Input: part model. Units: mm. Frame: model coordinates. Face numbers are marked on the shaded views. A direction names the side the tool comes from. Round coordinates to 2 decimals unless told otherwise and drop trailing zeros. Loops run counter-clockwise (first coordinate to the right, second up) from the corner with the lowest first, then second, coordinate; pieces in that order, holes last.
1) Section C-C, the plane y = 14.75. Return loops of the section in (x, z).
2) Section D-D, the plane z = 3.75. Return loops of the section in (x, y), and give its area (4 significant figures).
3) First-contact query: pin 1 (2.5 mm diameter, centred on x = 19.5, y = 4.5, fed in from +Z); pin 2 (8 mm diameter, centred on x = 25.5, y = 22, fed in from -Z); pin 3 (9.5 mm diameter, centred on x = 53.5, y = 13.5, fed in from +Z). Flat tips, straight axial feed; report the tip coordinate or a pass-through.
4) Section B-B, the plane x = 29. Return loops of the section in (y, z), and give its area (4 significant figures).
5) Draft query along X for the marked faces 1, 2 and 3. Return one class per face: pulls with the +X half, pulls with the -X half, needs draft (parallel to the pull), parting line crosses it, or undercut.
6) Section A-A, the plane z = 7.25. Return loops of the section in (x, y), and give its area (3 significant figures).
7) Access query for the marked faces 4, 5 and 6. Directions: +Z, -Z, +X, -X, +Y, -Y. A direction counts if a zero-diameter tool reaches every point of the face in a straight line with its end or side. Return the directions, or none.
8) Ray query, line 1 along Y through (x, z) = (57.5, 2.25); line 2 along Y through (x, z) = (41, 3.25); line 3 along X through (y, z) = (18.25, 4.5). Return the intervals inside material, ascending.
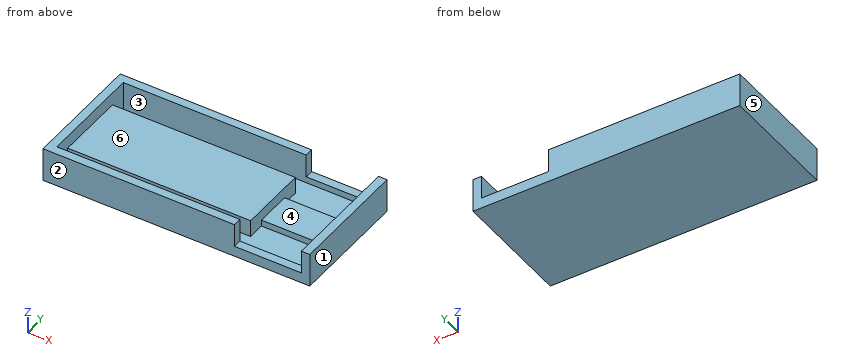
from build123d import *

# Parameters (mm, degrees)
F0_W     = 43.2
F0_H     = 4
F1_DEPTH = 1
F0_W_2   = 15.8
F0_H_2   = 2
F0_H_3   = 8.5
F2_DEPTH = 2.5
F3_DEPTH = 5
F4_DEPTH = 8


with BuildPart() as f1:
    # F0 (on Top) → F1 (new body)
    with BuildSketch(Plane.XY):
        Polygon((59, 16.5), (59, 24.5), (43.2, 24.5), (43.2, 20.5), (43.2, 16.5), align=None)
        with Locations((21.6, 22.5)):
            Rectangle(F0_W, F0_H)
    extrude(amount=F1_DEPTH)



with BuildPart() as f1b:
    # F0 (on Top) → F1, piece 2 (new body)
    with BuildSketch(Plane.XY):
        Polygon((59, 0), (59, 8), (43.2, 8), (43.2, 4), (43.2, 0), align=None)
        with Locations((21.6, 2)):
            Rectangle(F0_W, F0_H)
    extrude(amount=F1_DEPTH)


with BuildPart() as f1_1:
    add(f1.part)

    add(f1b.part)  # F2 merges F1b
    # F0 (on Top) → F2 (join)
    with BuildSketch(Plane.XY):
        with Locations((51.1, 25.5)):
            Rectangle(F0_W_2, F0_H_2)
        with Locations((51.1, 12.25)):
            Rectangle(F0_W_2, F0_H_3)
        with Locations((51.1, -1)):
            Rectangle(F0_W_2, F0_H_2)
    extrude(amount=F2_DEPTH)

    # F0 (on Top) → F3 (join)
    with BuildSketch(Plane.XY):
        Polygon((43.2, 8), (43.2, 16.5), (43.2, 20.5), (0, 20.5), (0, 4), (43.2, 4), align=None)
    extrude(amount=F3_DEPTH)

    # F0 (on Top) → F4 (join)
    with BuildSketch(Plane.XY):
        Polygon((43.2, 24.5), (43.2, 26.5), (-2, 26.5), (-2, -2), (43.2, -2), (43.2, 0), (0, 0), (0, 4), (0, 20.5), (0, 24.5), align=None)
        Polygon((61, 26.5), (59, 26.5), (59, 24.5), (59, 16.5), (59, 8), (59, 0), (59, -2), (61, -2), align=None)
    extrude(amount=F4_DEPTH)


solid = f1_1.part
Final values:
1. outline: (-2, 0) - (61, 0) - (61, 8) - (59, 8) - (59, 2.5) - (43.2, 2.5) - (43.2, 5) - (0, 5) - (0, 8) - (-2, 8) - close
2. outline: (-2, -2) - (43.2, -2) - (43.2, 0) - (0, 0) - (0, 4) - (43.2, 4) - (43.2, 20.5) - (0, 20.5) - (0, 24.5) - (43.2, 24.5) - (43.2, 26.5) - (-2, 26.5) - close; (59, -2) - (61, -2) - (61, 26.5) - (59, 26.5) - close
2. area: 1,000 mm2
3. pin 1: stops at z = 5
3. pin 2: stops at z = 0
3. pin 3: stops at z = 2.5
4. outline: (-2, 0) - (26.5, 0) - (26.5, 8) - (24.5, 8) - (24.5, 1) - (20.5, 1) - (20.5, 5) - (4, 5) - (4, 1) - (0, 1) - (0, 8) - (-2, 8) - close
4. area: 122.5 mm2
5. face 1: pulls with the +X half
5. face 2: needs draft
5. face 3: undercut
6. outline: (-2, -2) - (43.2, -2) - (43.2, 0) - (0, 0) - (0, 24.5) - (43.2, 24.5) - (43.2, 26.5) - (-2, 26.5) - close; (59, -2) - (61, -2) - (61, 26.5) - (59, 26.5) - close
6. area: 287 mm2
7. face 4: +Z, +Y, -Y
7. face 5: +Z, -Z, -X, +Y, -Y
7. face 6: +Z
8. line 1: y = -2 to 0, 8 to 16.5, 24.5 to 26.5
8. line 2: y = -2 to 0, 4 to 20.5, 24.5 to 26.5
8. line 3: x = -2 to 43.2, 59 to 61
